Design review of the part built by this model. Coordinates are the model's own, in mm. A direction names the side the tool comes from. Give positions to 0.01 mm unless a question says otherwise; leave off trailing zeros. Write each loop counter-clockwise with the first axis right and the second up, starting at its lowest first coordinate (ties: lowest second). Pieces come first, ordered by that corner, then holes.
```python
from build123d import *

# Parameters (mm, degrees)
SKETCH2_R          = 3
CUT_EXTRUDE1_DEPTH = 46.047530454


with BuildPart() as part:
    # Sketch1 → Revolve1 (revolve)
    with BuildSketch(Plane(origin=(0, 0, 0), x_dir=(0, 0, -1), z_dir=(1, 0, 0)), mode=Mode.PRIVATE) as revolve1_sk:
        Polygon((-3, 0), (-28.4, 0), (-28.4, 6), (-15, 6), (-15, 26.4), (-3, 26.4), align=None)
    revolve(revolve1_sk.sketch.rotate(Axis((0, 0, 0), (0, 1, 0)), 180), axis=Axis((0, 0, 0), (0, 1, 0)))

    # Sketch2 → Cut-Extrude1 (cut, through all)
    with BuildSketch(Plane(origin=(0, 6, 0), x_dir=(1, 0, 0), z_dir=(0, 1, 0))):
        with Locations(Location((0, 23.75, 0), (0, 0, 270))):
            Circle(SKETCH2_R)
        with Locations(Location((20.56810334, 11.875, 0), (0, 0, 270))):
            Circle(SKETCH2_R)
        with Locations(Location((20.56810334, -11.875, 0), (0, 0, 270))):
            Circle(SKETCH2_R)
        with Locations(Location((0, -23.75, 0), (0, 0, 270))):
            Circle(SKETCH2_R)
        with Locations(Location((-20.56810334, -11.875, 0), (0, 0, 270))):
            Circle(SKETCH2_R)
        with Locations(Location((-20.56810334, 11.875, 0), (0, 0, 270))):
            Circle(SKETCH2_R)
    extrude(amount=-CUT_EXTRUDE1_DEPTH, mode=Mode.SUBTRACT)


solid = part.part
```
(1) Consider section D-D, the plane y = 13. Give the boundary of the cut face in (x, z), then the cut area to 3 significant figures.
Resolved:
outline: circle Ø30 at (0, 0); hole circle Ø6 at (0, 0)
area: 679 mm2
(2) Clearance check with flat-ended pins moving along their axes: P1, Ø4, axis at y = 10.5, z = -15, coming from the -X side; P2, Ø8, axis at y = 19, z = 15.5, coming from the +X side; P3, Ø9.5, axis at x = -20.57, z = 11.88, coming from the +Y side. State where each tip first meets the part, or that it passes through.
Resolved:
P1: stops at x = -7.48
P2: stops at x = 9.63
P3: stops at y = 6
(3) To check wall thickness, follow L1, parallel to X at y = 7, z = 0; L2, parallel to Y at x = 14, z = -17; L3, parallel to X at y = 1.75, z = 24. State the ranges of each line that lie inside material, in increasing order.
Resolved:
L1: x = -15 to -3, 3 to 15
L2: y = 0 to 6
L3: x = -15.18 to -2.99, 2.99 to 15.18
(4) Consider section C-C, the plane y = 5. Give the boundary of the cut face in (x, z) (3 decimals), then the cut area to 3 significant figures.
Resolved:
outline: circle Ø56.8 at (0, 0); hole circle Ø6 at (-20.568, -11.875); hole circle Ø6 at (-20.568, 11.875); hole circle Ø6 at (0, -23.75); hole circle Ø6 at (0, 0); hole circle Ø6 at (0, 23.75); hole circle Ø6 at (20.568, -11.875); hole circle Ø6 at (20.568, 11.875)
area: 2,340 mm2
(5) Mouldability with a two-part tool opening along Z and no side actions: class faces 1 (the face through (-18.5, 3, 9.7)), 2 (the face through (-12.65, 16.34, -8.06)), 3 (the face through (18.743, 3.042, -14.256)), 4 (the face through (0, 0, 6)) as pulls with the +Z half, pulls with the -Z half, needs draft (parallel to the pull), parting line crosses it, or undercut.
Resolved:
face 1: undercut
face 2: parting line crosses it
face 3: undercut
face 4: needs draft
(6) Consider section A-A, the plane x = 0. Give the boundary of the cut face in (y, z).
Resolved:
outline: (0, -28.4) - (6, -28.4) - (6, -26.75) - (0, -26.75) - close; (0, -20.75) - (6, -20.75) - (6, -15) - (26.4, -15) - (26.4, -3) - (0, -3) - close; (0, 3) - (26.4, 3) - (26.4, 15) - (6, 15) - (6, 20.75) - (0, 20.75) - close; (0, 26.75) - (6, 26.75) - (6, 28.4) - (0, 28.4) - close
(7) Consider section B-B, the plane z = -23.75. Give the boundary of the cut face in (x, y), then the cut area to 3 significant figures.
Resolved:
outline: (-15.57, 0) - (-3, 0) - (-3, 6) - (-15.57, 6) - close; (3, 0) - (15.57, 0) - (15.57, 6) - (3, 6) - close
area: 151 mm2
(8) Tool access review of faces 5 (the face through (0.132, 3.042, -26.747)), 6 (the face through (12, 6, -12)): name each direction out of +Z, -Z, +X, -X, +Y, -Y from which nothing blocks a thin tool from reaching the whole face with its end or side.
Resolved:
face 5: +Y, -Y
face 6: +Y
